Design review of the part built by this model. Coordinates are the model's own, in mm. Give positions to 0.01 mm unless a question says otherwise; leave off trailing zeros.
```python
from build123d import *

# Parameters (mm, degrees)
F0_R     = 6.35
F0_R_2   = 4.7625
F1_DEPTH = 63.5
F2_SIZE  = 0.635


with BuildPart() as f1:
    # F0 (on Top) → F1 (new body)
    with BuildSketch(Plane.XY):
        Circle(F0_R)
        Circle(F0_R_2, mode=Mode.SUBTRACT)
    extrude(amount=F1_DEPTH)

    # F2
    f2_edges = [f1.edges().sort_by_distance(p)[0] for p in [
        (6.35, 0, 31.75),
        (-6.35, 0, 0),
        (-6.35, 0, 63.5),
        (4.7625, 0, 31.75),
        (-4.7625, 0, 0),
        (-4.7625, 0, 63.5),
    ]]
    chamfer(f2_edges, length=F2_SIZE)


solid = f1.part
```
(1) To check wall thickness, follow L1, parallel to Y at x = 0, z = 30; L2, parallel to X at y = 2.5, z = 23.5; L3, parallel to Y at x = -3.25, z = 36. State the ranges of each line that lie inside material, in increasing order.
Resolved:
L1: y = -6.35 to -4.76, 4.76 to 6.35
L2: x = -5.84 to -4.05, 4.05 to 5.84
L3: y = -5.46 to -3.48, 3.48 to 5.46
(2) Mouldability with a two-part tool opening along X and no side actions: class faces 1 (the face through (-1.38, -6.2, 31.31)), 2 (the face through (-3.78, -2.9, 31.31)) as pulls with the +X half, pulls with the -X half, needs draft (parallel to the pull), parting line crosses it, or undercut.
Resolved:
face 1: parting line crosses it
face 2: undercut
(3) Clearance check with flat-ended pins moving along their axes: P1, Ø1, axis at y = -1.5, z = 23.5, coming from the +X side; P2, Ø1.5, axis at x = 4.5, y = 0.5, coming from the -Z side; P3, Ø1, axis at x = 3.5, y = 3, coming from the -Z side; P4, Ø6, axis at x = -2, z = 23.5, coming from the +Y side. State where each tip first meets the part, or that it passes through.
Resolved:
P1: stops at x = 6.27
P2: stops at z = 0.12
P3: stops at z = 0.29
P4: stops at y = 6.35
